Input: part model. Units: mm. Frame: model coordinates. Face numbers are marked on the shaded views. A direction names the side the tool comes from. Round coordinates to 2 decimals unless told otherwise and drop trailing zeros. Loops run counter-clockwise (first coordinate to the right, second up) from the corner with the lowest first, then second, coordinate; pieces in that order, holes last.
1) Section A-A, the plane z = 11. Return loops of the section in (x, y), and give its area (3 significant figures).
2) Section D-D, the plane x = 0. Return loops of the section in (y, z), and give its area (3 significant figures).
3) Ray query, line 1 along Y through (x, z) = (0, 7.5); line 2 along Y through (x, z) = (0, 12.3); line 3 along Y through (x, z) = (0, 10.25). Return the intervals inside material, ascending.
4) Section B-B, the plane z = 5.5. State how many separate pieces and enclosed holes the cut face has, and give its area (3 significant figures).
5) Section C-C, the plane y = 0. Return loops of the section in (x, z), and give its area (3 significant figures).
6) First-contact query: pin 1 (2.5 mm diameter, centred on x = -4, z = 5, fed in from -Y); pin 2 (1 mm diameter, centred on x = 3.5, z = 2, fed in from -Y); pin 3 (3 mm diameter, centred on y = -10, z = 12.5, fed in from -X); pin 4 (6 mm diameter, centred on x = -0.5, z = 3, fed in from -Y). Flat tips, straight axial feed; report the tip coordinate or a pass-through.
7) Draft query along X for the marked faces 3, 4 and 5. Return one class per face: pulls with the +X half, pulls with the -X half, needs draft (parallel to the pull), parting line crosses it, or undercut.
8) Access query for the marked faces 1 and 2. Directions: +Z, -Z, +X, -X, +Y, -Y. A direction counts if a zero-diameter tool reaches every point of the face in a straight line with its end or side. Return the directions, or none.
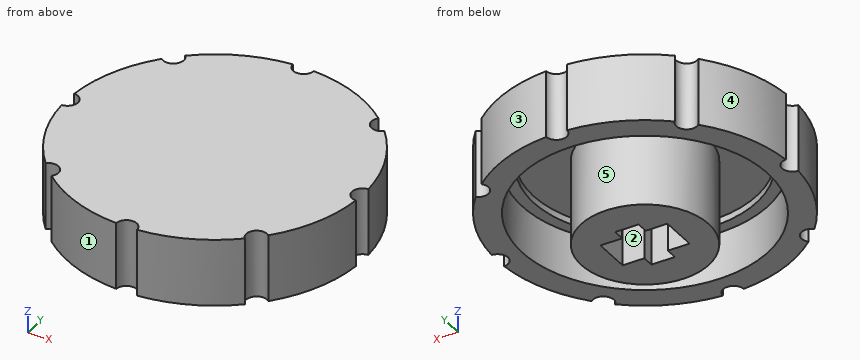
from build123d import *

# Parameters (mm, degrees)
SKETCH004_W        = 3.5
SKETCH004_H        = 9
POCKET001_DEPTH    = 8
SKETCH005_W        = 10
SKETCH005_H        = 5.5
POCKET002_DEPTH    = 7
SKETCH007_R        = 1.55
POCKET003_DEPTH    = 142.723477
POLARPATTERN_COUNT = 8


with BuildPart() as part:
    # Sketch → Revolution (revolve)
    with BuildSketch(Plane.XZ):
        Polygon((-18.3, 4.8), (-22, 4.8), (-22, 14.8), (0, 14.8), (0, 0), (-9.5, 0), (-9.5, 12.8), (-16.6, 12.8), (-16.6, 11.8), (-18.3, 11.8), align=None)
    revolve(axis=Axis((0, 0, 0), (0, 0, 1)))

    # Sketch004 (on Face4 of Revolution) → Pocket001 (cut)
    with BuildSketch(Plane(origin=(0, 0, 0), x_dir=(1, 0, 0), z_dir=(0, 0, -1))):
        Rectangle(SKETCH004_W, SKETCH004_H)
    extrude(amount=-POCKET001_DEPTH, mode=Mode.SUBTRACT)

    # Sketch005 (on Face9 of Pocket001) → Pocket002 (cut)
    with BuildSketch(Plane(origin=(0, 0, 0), x_dir=(1, 0, 0), z_dir=(0, 0, -1))):
        Rectangle(SKETCH005_W, SKETCH005_H)
    extrude(amount=-POCKET002_DEPTH, mode=Mode.SUBTRACT)

    # Sketch007 (on Face5 of Pocket002) → Pocket003 (cut, through all)
    with BuildSketch(Plane(origin=(0, 0, 14.8), x_dir=(-1, 0, 0), z_dir=(0, 0, 1))):
        with Locations((-22, 0)):
            Circle(SKETCH007_R)
    pocket003 = extrude(amount=-POCKET003_DEPTH, mode=Mode.SUBTRACT)

    # PolarPattern: Pocket003 ×8 about axis
    polarpattern_axis = Axis((0, 0, 0), (0, 0, 1))
    for i in range(1, POLARPATTERN_COUNT):
        add(pocket003.rotate(polarpattern_axis, i * 360 / POLARPATTERN_COUNT), mode=Mode.SUBTRACT)


solid = part.part
Final values:
1. outline: (-21.95, -1.55) arc R22 ccw to (-16.61, -14.42) arc R1.55 cw to (-14.42, -16.61) arc R22 ccw to (-1.55, -21.95) arc R1.55 cw to (1.55, -21.95) arc R22 ccw to (14.42, -16.61) arc R1.55 cw to (16.61, -14.42) arc R22 ccw to (21.95, -1.55) arc R1.55 cw to (21.95, 1.55) arc R22 ccw to (16.61, 14.42) arc R1.55 cw to (14.42, 16.61) arc R22 ccw to (1.55, 21.95) arc R1.55 cw to (-1.55, 21.95) arc R22 ccw to (-14.42, 16.61) arc R1.55 cw to (-16.61, 14.42) arc R22 ccw to (-21.95, 1.55) arc R1.55 cw to start; circle Ø19 at (0, 0); hole circle Ø36.6 at (0, 0)
1. area: 722 mm2
2. outline: (-20.45, 4.8) - (-18.3, 4.8) - (-18.3, 11.8) - (-16.6, 11.8) - (-16.6, 12.8) - (-9.5, 12.8) - (-9.5, 0) - (-4.5, 0) - (-4.5, 8) - (4.5, 8) - (4.5, 0) - (9.5, 0) - (9.5, 12.8) - (16.6, 12.8) - (16.6, 11.8) - (18.3, 11.8) - (18.3, 4.8) - (20.45, 4.8) - (20.45, 14.8) - (-20.45, 14.8) - close
2. area: 291 mm2
3. line 1: y = -20.45 to -18.3, -9.5 to -4.5, 4.5 to 9.5, 18.3 to 20.45
3. line 2: y = -20.45 to -16.6, -9.5 to 9.5, 16.6 to 20.45
3. line 3: y = -20.45 to -18.3, -9.5 to 9.5, 18.3 to 20.45
4. separate pieces: 2
4. enclosed holes: 2
4. area: 655 mm2
5. outline: (-20.45, 4.8) - (-18.3, 4.8) - (-18.3, 11.8) - (-16.6, 11.8) - (-16.6, 12.8) - (-9.5, 12.8) - (-9.5, 0) - (-5, 0) - (-5, 7) - (-1.75, 7) - (-1.75, 8) - (1.75, 8) - (1.75, 7) - (5, 7) - (5, 0) - (9.5, 0) - (9.5, 12.8) - (16.6, 12.8) - (16.6, 11.8) - (18.3, 11.8) - (18.3, 4.8) - (20.45, 4.8) - (20.45, 14.8) - (-20.45, 14.8) - close
5. area: 289 mm2
6. pin 1: stops at y = -21.83
6. pin 2: stops at y = -9.01
6. pin 3: stops at x = -20.29
6. pin 4: stops at y = -21.95
7. face 3: pulls with the +X half
7. face 4: pulls with the -X half
7. face 5: undercut
8. face 1: +Z, -Z, -X, -Y
8. face 2: -Z
